The drawing under review shows one solid part. Ordinate dimensions are in mm from its lowest x, y, z. A direction names the side the tool comes from. Coordinates: 2 decimals unless noted, no trailing zeros. Write each loop counter-clockwise with the first axis right and the second up, starting at its lowest first coordinate (ties: lowest second). Pieces come first, ordered by that corner, then holes. Notation, with made-up numbers: (12, 16) - (40, 16) arc R15 cw to (40, 36) - close; hole circle Ø10 at (-13.75, 61.5). An arc over 180 degrees is marked (long way). Use a Markdown table: item, result.
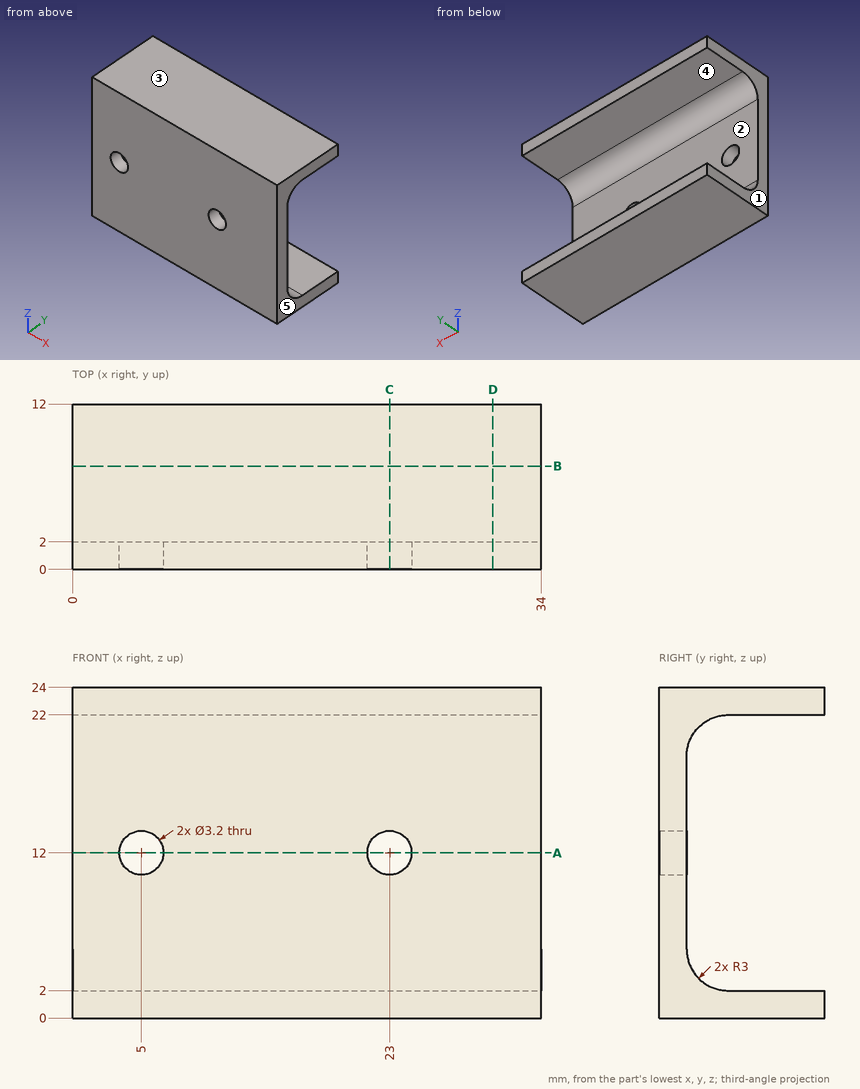
(1) Machinability: for the marked faces 1 and 2, which of the approach directions +Z, -Z, +X, -X, +Y, -Y give a long, thin tool a straight path to every point of the face, cutting with its end or side? Answer none if there is none.
Determined:
| item | result |
|---|---|
| face 1 | +Z, -Z, -X, +Y, -Y |
| face 2 | +X, -X, +Y |
(2) Take a section at D-D on x = 30.5. Write out the cut boundary in (y, z).
Determined:
| item | result |
|---|---|
| outline | (0, 0) - (12, 0) - (12, 2) - (5, 2) arc R3 cw to (2, 5) - (2, 19) arc R3 cw to (5, 22) - (12, 22) - (12, 24) - (0, 24) - close |
(3) Take a section at C-C on x = 23. Write out the cut boundary in (y, z), and give its area (3 significant figures).
Determined:
| item | result |
|---|---|
| outline | (0, 0) - (12, 0) - (12, 2) - (5, 2) arc R3 cw to (2, 5) - (2, 10.4) - (0, 10.4) - close; (0, 13.6) - (2, 13.6) - (2, 19) arc R3 cw to (5, 22) - (12, 22) - (12, 24) - (0, 24) - close |
| area | 85.5 mm2 |
(4) Take a section at A-A on z = 12. Write out the cut boundary in (x, y).
Determined:
| item | result |
|---|---|
| outline | (0, 0) - (3.4, 0) - (3.4, 2) - (0, 2) - close; (6.6, 0) - (21.4, 0) - (21.4, 2) - (6.6, 2) - close; (24.6, 0) - (34, 0) - (34, 2) - (24.6, 2) - close |
(5) For pin 1 (4 mm diameter, centred on x = 23, z = 12, fed in from +Y); pin 2 (1.5 mm diameter, centred on x = 26.5, z = 4.5, fed in from +Y), all flat-tipped, find the tip position at first contact; note any pin that passes through.
Determined:
| item | result |
|---|---|
| pin 1 | y = 2 |
| pin 2 | y = 2.27 |
(6) For L1, parallel to X at y = 0.6, z = 12; L2, parallel to Z at x = 23, y = 1.1; L3, parallel to Z at x = 8, y = 7, list the stretches that pass through material, from the lowest coordinate up. Write a range as from..to.
Determined:
| item | result |
|---|---|
| L1 | 0..3.4, 6.6..21.4, 24.6..34 |
| L2 | 0..10.4, 13.6..24 |
| L3 | 0..2, 22..24 |
(7) Take a section at B-B on y = 7.5. Write out the cut boundary in (x, z).
Determined:
| item | result |
|---|---|
| outline | (0, 0) - (34, 0) - (34, 2) - (0, 2) - close; (0, 22) - (34, 22) - (34, 24) - (0, 24) - close |
(8) Draft analysis for pull direction Z (two halves, no side actions). For the marked faces 3, 4 and 5, state which applies: +Z half, -Z half, draft (parallel to the pull), parting line (faces both ways), or undercut.
Determined:
| item | result |
|---|---|
| face 3 | +Z half |
| face 4 | undercut |
| face 5 | draft |
